```python
from build123d import *

# Parameters (mm, degrees)
SZKIC1_W                    = 20
SZKIC1_H                    = 12
SZKIC1_R                    = 5
DODANIE_WYCI_GNI_CIE1_DEPTH = 15
OTW_R_3_2_3_2_1_D           = 3.2


with BuildPart() as part:
    # Szkic1 → Dodanie-wyciągnięcie1 (new body)
    with BuildSketch(Plane(origin=(0, 0, 0), x_dir=(1, 0, 0), z_dir=(0, 1, 0))):
        Rectangle(SZKIC1_W, SZKIC1_H)
        with Locations(Location((0, 0, 0), (0, 0, 270))):
            Circle(SZKIC1_R, mode=Mode.SUBTRACT)
    extrude(amount=DODANIE_WYCI_GNI_CIE1_DEPTH)

    # Otwór Ø3.2 (3.2)1 (through all)
    with Locations(Plane.XY.offset(6)):
        with Locations((8, 12.5), (-8, 12.5), (-8, 2.5), (8, 2.5)):
            Hole(OTW_R_3_2_3_2_1_D / 2)


solid = part.part
```
Here's how the part is built. I have some questions about the finished solid (model axes, mm). Give positions to 0.01 mm unless a question says otherwise; leave off trailing zeros. Loops run counter-clockwise (first coordinate to the right, second up) from the corner with the lowest first, then second, coordinate; pieces in that order, holes last. Notation, with made-up numbers: M 52,-2 L 65,-2 A18 cw 65,3 Z; hole C -23.5,-7.75 d8. An arc over 180 degrees is marked long. Use one line per item in the form item = value. Start each with the question number.
Q1. Thinking about a two-plate mould opening in Y: for faces 1 (the cylindrical face through (-6.82, 13.58, -0.08)), 2 (the cylindrical face through (-6.4, 2.57, -0.08)), 3 (the cylindrical face through (-4.88, 7.4, -1.08)), 4 (the flat face through (-5, 15, 3)), which applies, +Y half, -Y half, draft (parallel to the pull), parting line (faces both ways), or undercut?
Q2. If we section it at B-B (z = 0): Write out the boundary of the cut face in (x, y), then the cut area to 3 significant figures.
Q3. If we section it at D-D (x = 2.25): Write out the boundary of the cut face in (y, z), then the cut area to 3 significant figures.
Q4. I need wall thicknesses on line 1 along Y through (x, z) = (-8, 3.75); line 2 along X through (y, z) = (12.25, 1.25); line 3 along X through (y, z) = (8.75, 0). Which ranges of each line are inside material? Lowest first, please.
Q5. If we section it at A-A (x = 8): Write out the boundary of the cut face in (y, z), then the cut area to 3 significant figures.
Q6. If we section it at C-C (y = 2.5): Write out the boundary of the cut face in (x, z), then the cut area to 3 significant figures.
Q7. Will this pin go through, and if not, where does the flat tip stop? pin 1 Ø3 at (x, y) = (-8, 12.5) entering from +Z.
Taken from the geometry:
q1.face_1 = undercut
q1.face_2 = undercut
q1.face_3 = draft
q1.face_4 = +Y half
q2.outline = M -10,0 L -5,0 L -5,15 L -10,15 Z; M 5,0 L 10,0 L 10,15 L 5,15 Z; hole C -8,2.5 d3.2; hole C -8,12.5 d3.2; hole C 8,2.5 d3.2; hole C 8,12.5 d3.2
q2.area = 118 mm^2
q3.outline = M 0,-6 L 15,-6 L 15,-4.47 L 0,-4.47 Z; M 0,4.47 L 15,4.47 L 15,6 L 0,6 Z
q3.area = 46.0 mm^2
q4.line_1 = 0 to 0.9, 4.1 to 10.9, 14.1 to 15
q4.line_2 = -10 to -9.58, -6.42 to -4.84, 4.84 to 6.42, 9.58 to 10
q4.line_3 = -10 to -5, 5 to 10
q5.outline = M 0,-6 L 0.9,-6 L 0.9,6 L 0,6 Z; M 4.1,-6 L 10.9,-6 L 10.9,6 L 4.1,6 Z; M 14.1,-6 L 15,-6 L 15,6 L 14.1,6 Z
q5.area = 103 mm^2
q6.outline = M -10,-6 L -9.6,-6 L -9.6,6 L -10,6 Z; M -6.4,-6 L 6.4,-6 L 6.4,6 L -6.4,6 Z; M 9.6,-6 L 10,-6 L 10,6 L 9.6,6 Z; hole C 0,0 d10
q6.area = 84.7 mm^2
q7.pin_1 = through
